Geometry check sheet. Reference: the model listing, model coordinates, mm. Face numbers are marked on the shaded views. A direction names the side the tool comes from. Coordinates: 2 decimals unless noted, no trailing zeros. Answer as CSV lines item,"result".
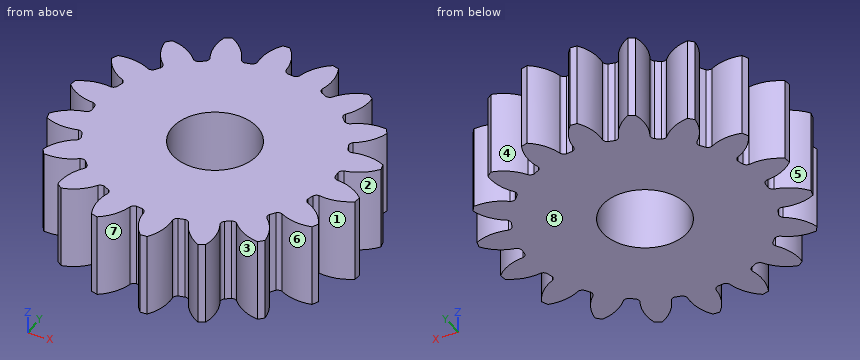
```python
from build123d import *

# Parameters (mm, degrees)
F0_R     = 5
F1_DEPTH = 10


with BuildPart() as f1:
    # F0 (on Top) → F1 (new body)
    with BuildSketch(Plane.XY):
        with BuildLine():
            ThreePointArc((0.834247, 13.754724), (0.539473, 13.922611), (0.384061, 14.224148))
            ThreePointArc((0.384061, 14.224148), (-0.053041, 16.126356), (-1.146638, 17.742988))
            Line((-1.146638, 17.742988), (-1.950006, 17.672744))
            ThreePointArc((-1.950006, 17.672744), (-2.74627, 15.891587), (-2.846993, 13.943148))
            ThreePointArc((-2.846993, 13.943148), (-2.94723, 13.618388), (-3.20868, 13.401223))
            Line((-3.20868, 13.401223), (-3.920457, 13.210542))
            ThreePointArc((-3.920457, 13.210542), (-4.254874, 13.267486), (-4.504046, 13.497684))
            ThreePointArc((-4.504046, 13.497684), (-5.565381, 15.135677), (-7.145946, 16.280782))
            Line((-7.145946, 16.280782), (-7.876841, 15.940006))
            ThreePointArc((-7.876841, 15.940006), (-8.015892, 13.993927), (-7.444136, 12.128545))
            ThreePointArc((-7.444136, 12.128545), (-7.427254, 11.789086), (-7.598661, 11.495597))
            Line((-7.598661, 11.495597), (-8.202296, 11.072974))
            ThreePointArc((-8.202296, 11.072974), (-8.536021, 11.012106), (-8.848898, 11.1432))
            ThreePointArc((-8.848898, 11.1432), (-10.406453, 12.319412), (-12.283348, 12.854873))
            Line((-12.283348, 12.854873), (-12.853612, 12.284668))
            ThreePointArc((-12.853612, 12.284668), (-12.31868, 10.408393), (-11.143406, 8.85106))
            ThreePointArc((-11.143406, 8.85106), (-11.01144, 8.537847), (-11.072132, 8.203432))
            Line((-11.072132, 8.203432), (-11.494817, 7.599841))
            ThreePointArc((-11.494817, 7.599841), (-11.787598, 7.428503), (-12.126443, 7.444681))
            ThreePointArc((-12.126443, 7.444681), (-13.992354, 8.017243), (-15.939197, 7.878477))
            Line((-15.939197, 7.878477), (-16.280048, 7.147617))
            ThreePointArc((-16.280048, 7.147617), (-15.135653, 5.567454), (-13.498617, 4.506006))
            ThreePointArc((-13.498617, 4.506006), (-13.267485, 4.256818), (-13.21014, 3.921813))
            Line((-13.21014, 3.921813), (-13.400893, 3.210056))
            ThreePointArc((-13.400893, 3.210056), (-13.617417, 2.948914), (-13.94136, 2.848224))
            ThreePointArc((-13.94136, 2.848224), (-15.890571, 2.748077), (-17.672544, 1.95182))
            Line((-17.672544, 1.95182), (-17.74287, 1.148459))
            ThreePointArc((-17.74287, 1.148459), (-16.127043, 0.054997), (-14.225696, -0.382538))
            ThreePointArc((-14.225696, -0.382538), (-13.923275, -0.537647), (-13.75481, -0.832836))
            Line((-13.75481, -0.832836), (-13.690624, -1.566909))
            ThreePointArc((-13.690624, -1.566909), (-13.804774, -1.886358), (-14.074743, -2.091771))
            ThreePointArc((-14.074743, -2.091771), (-15.87215, -2.852547), (-17.274321, -4.210255))
            Line((-17.274321, -4.210255), (-17.06564, -4.989221))
            ThreePointArc((-17.06564, -4.989221), (-15.173273, -5.464093), (-13.236946, -5.224943))
            ThreePointArc((-13.236946, -5.224943), (-12.899713, -5.267264), (-12.640446, -5.487031))
            Line((-12.640446, -5.487031), (-12.329064, -6.154883))
            ThreePointArc((-12.329064, -6.154883), (-12.327072, -6.494108), (-12.510505, -6.779467))
            ThreePointArc((-12.510505, -6.779467), (-13.939314, -8.109113), (-14.79256, -9.864511))
            Line((-14.79256, -9.864511), (-14.330042, -10.525127))
            ThreePointArc((-14.330042, -10.525127), (-12.389383, -10.324133), (-10.651624, -9.437142))
            ThreePointArc((-10.651624, -9.437142), (-10.320255, -9.36157), (-10.001459, -9.47941))
            Line((-10.001459, -9.47941), (-9.480437, -10.000486))
            ThreePointArc((-9.480437, -10.000486), (-9.362542, -10.318572), (-9.437314, -10.64946))
            ThreePointArc((-9.437314, -10.64946), (-10.32519, -12.387599), (-10.526598, -14.328962))
            Line((-10.526598, -14.328962), (-9.86603, -14.791547))
            ThreePointArc((-9.86603, -14.791547), (-8.11115, -13.93893), (-6.78156, -12.511083))
            ThreePointArc((-6.78156, -12.511083), (-6.496022, -12.326734), (-6.156148, -12.328432))
            Line((-6.156148, -12.328432), (-5.488329, -12.639883))
            ThreePointArc((-5.488329, -12.639883), (-5.268753, -12.898464), (-5.225845, -13.234971))
            ThreePointArc((-5.225845, -13.234971), (-5.465697, -15.171959), (-4.990972, -17.065128))
            Line((-4.990972, -17.065128), (-4.212028, -17.273888))
            ThreePointArc((-4.212028, -17.273888), (-2.854593, -15.872486), (-2.093539, -14.076003))
            ThreePointArc((-2.093539, -14.076003), (-1.888272, -13.805111), (-1.568315, -13.690463))
            Line((-1.568315, -13.690463), (-0.834247, -13.754724))
            ThreePointArc((-0.834247, -13.754724), (-0.539473, -13.922611), (-0.384061, -14.224148))
            ThreePointArc((-0.384061, -14.224148), (0.053041, -16.126356), (1.146638, -17.742988))
            Line((1.146638, -17.742988), (1.950006, -17.672744))
            ThreePointArc((1.950006, -17.672744), (2.74627, -15.891587), (2.846993, -13.943148))
            ThreePointArc((2.846993, -13.943148), (2.94723, -13.618388), (3.20868, -13.401223))
            Line((3.20868, -13.401223), (3.920457, -13.210542))
            ThreePointArc((3.920457, -13.210542), (4.254874, -13.267486), (4.504046, -13.497684))
            ThreePointArc((4.504046, -13.497684), (5.565381, -15.135677), (7.145946, -16.280782))
            Line((7.145946, -16.280782), (7.876841, -15.940006))
            ThreePointArc((7.876841, -15.940006), (8.015892, -13.993927), (7.444136, -12.128545))
            ThreePointArc((7.444136, -12.128545), (7.427254, -11.789086), (7.598661, -11.495597))
            Line((7.598661, -11.495597), (8.202296, -11.072974))
            ThreePointArc((8.202296, -11.072974), (8.536021, -11.012106), (8.848898, -11.1432))
            ThreePointArc((8.848898, -11.1432), (10.406453, -12.319412), (12.283348, -12.854873))
            Line((12.283348, -12.854873), (12.853612, -12.284668))
            ThreePointArc((12.853612, -12.284668), (12.31868, -10.408393), (11.143406, -8.85106))
            ThreePointArc((11.143406, -8.85106), (11.01144, -8.537847), (11.072132, -8.203432))
            Line((11.072132, -8.203432), (11.494817, -7.599841))
            ThreePointArc((11.494817, -7.599841), (11.787598, -7.428503), (12.126443, -7.444681))
            ThreePointArc((12.126443, -7.444681), (13.992354, -8.017243), (15.939197, -7.878477))
            Line((15.939197, -7.878477), (16.280048, -7.147617))
            ThreePointArc((16.280048, -7.147617), (15.135653, -5.567454), (13.498617, -4.506006))
            ThreePointArc((13.498617, -4.506006), (13.267485, -4.256818), (13.21014, -3.921813))
            Line((13.21014, -3.921813), (13.400893, -3.210056))
            ThreePointArc((13.400893, -3.210056), (13.617417, -2.948914), (13.94136, -2.848224))
            ThreePointArc((13.94136, -2.848224), (15.890571, -2.748077), (17.672544, -1.95182))
            Line((17.672544, -1.95182), (17.74287, -1.148459))
            ThreePointArc((17.74287, -1.148459), (16.127043, -0.054997), (14.225696, 0.382538))
            ThreePointArc((14.225696, 0.382538), (13.923275, 0.537647), (13.75481, 0.832836))
            Line((13.75481, 0.832836), (13.690624, 1.566909))
            ThreePointArc((13.690624, 1.566909), (13.804774, 1.886358), (14.074743, 2.091771))
            ThreePointArc((14.074743, 2.091771), (15.87215, 2.852547), (17.274321, 4.210255))
            Line((17.274321, 4.210255), (17.06564, 4.989221))
            ThreePointArc((17.06564, 4.989221), (15.173273, 5.464093), (13.236946, 5.224943))
            ThreePointArc((13.236946, 5.224943), (12.899713, 5.267264), (12.640446, 5.487031))
            Line((12.640446, 5.487031), (12.329064, 6.154883))
            ThreePointArc((12.329064, 6.154883), (12.327072, 6.494108), (12.510505, 6.779467))
            ThreePointArc((12.510505, 6.779467), (13.939314, 8.109113), (14.79256, 9.864511))
            Line((14.79256, 9.864511), (14.330042, 10.525127))
            ThreePointArc((14.330042, 10.525127), (12.389383, 10.324133), (10.651624, 9.437142))
            ThreePointArc((10.651624, 9.437142), (10.320255, 9.36157), (10.001459, 9.47941))
            Line((10.001459, 9.47941), (9.480437, 10.000486))
            ThreePointArc((9.480437, 10.000486), (9.362542, 10.318572), (9.437314, 10.64946))
            ThreePointArc((9.437314, 10.64946), (10.32519, 12.387599), (10.526598, 14.328962))
            Line((10.526598, 14.328962), (9.86603, 14.791547))
            ThreePointArc((9.86603, 14.791547), (8.11115, 13.93893), (6.78156, 12.511083))
            ThreePointArc((6.78156, 12.511083), (6.496022, 12.326734), (6.156148, 12.328432))
            Line((6.156148, 12.328432), (5.488329, 12.639883))
            ThreePointArc((5.488329, 12.639883), (5.268753, 12.898464), (5.225845, 13.234971))
            ThreePointArc((5.225845, 13.234971), (5.465697, 15.171959), (4.990972, 17.065128))
            Line((4.990972, 17.065128), (4.212028, 17.273888))
            ThreePointArc((4.212028, 17.273888), (2.854593, 15.872486), (2.093539, 14.076003))
            ThreePointArc((2.093539, 14.076003), (1.888272, 13.805111), (1.568315, 13.690463))
            Line((1.568315, 13.690463), (0.834247, 13.754724))
        make_face()
        Circle(F0_R, mode=Mode.SUBTRACT)
    extrude(amount=F1_DEPTH)


solid = f1.part
```
Item 1: Depth check by flat-ended pin: pin 1 Ø6 at (y, z) = (6, 3.5) entering from +X; pin 2 Ø6 at (x, y) = (0, 0) entering from -Z; pin 3 Ø4 at (y, z) = (4.5, 4) entering from -X; pin 4 Ø4 at (x, z) = (6.5, 5) entering from +Y. Enter the tip coordinate at first touch or a pass-through.
Responses:
pin 1,"stops at x = 17.27"
pin 2,"passes through"
pin 3,"stops at x = -16.66"
pin 4,"stops at y = 17.2"
Item 2: Thickness scan on probe 1 along Y at (x, z) = (-15, 4); probe 2 along Y at (x, z) = (14.5, 2.75); probe 3 along Y at (x, z) = (0, 4.5). Record the ranges inside material, lowest first.
Responses:
probe 1,"y = -5.47 to -2.39, -0.29 to 2.88, 5.44 to 8.04"
probe 2,"y = -8.05 to -5.05, -2.89 to 0.36, 2.2 to 5.46, 9.06 to 10.28"
probe 3,"y = -16 to -5, 5 to 16"
Item 3: Set-up check for the marked faces 1, 2, 3, 4 and 5: record each of +Z, -Z, +X, -X, +Y, -Y from which the full face is reachable in a straight line by a thin tool's end or side.
Responses:
face 1,"+Z, -Z"
face 2,"+Z, -Z, +X"
face 3,"+Z, -Z, -Y"
face 4,"+Z, -Z, +Y"
face 5,"+Z, -Z, -X"
Item 4: Release check for a two-part mould opening along Y. For the marked faces 6, 7 and 8 record: +Y half, -Y half, draft (parallel to the pull), parting line (faces both ways), or undercut.
Responses:
face 6,"undercut"
face 7,"-Y half"
face 8,"draft"
